Here's how the part is built. I have some questions about the finished solid (model axes, mm). Give positions to 0.01 mm unless a question says otherwise; leave off trailing zeros. Write each loop counter-clockwise with the first axis right and the second up, starting at its lowest first coordinate (ties: lowest second). Pieces come first, ordered by that corner, then holes. Notation, with made-up numbers: (8.25, -3.5) -> (19.25, -3.5) arc R23 ccw to (19.25, 13.5) -> close; hole circle Ø8 at (59, 38). An arc over 180 degrees is marked (long way). Use one line per item in the form item = value.
```python
from build123d import *

# Parameters (mm, degrees)
SKETCH1_W             = 38.1
SKETCH1_H             = 9.525
BOSS_EXTRUDE1_DEPTH   = 6.35
F_4_CLEARANCE_HOLE1_D = 3.2639


with BuildPart() as part:
    # Sketch1 → Boss-Extrude1 (new body)
    with BuildSketch(Plane(origin=(0, 0, 0), x_dir=(1, 0, 0), z_dir=(0, 1, 0))):
        Rectangle(SKETCH1_W, SKETCH1_H)
    extrude(amount=BOSS_EXTRUDE1_DEPTH)

    # #4 Clearance Hole1 (through all)
    with Locations(Plane(origin=(0, 6.35, 0), x_dir=(1, 0, 0), z_dir=(0, 1, 0))):
        with Locations((-14.2875, 0)):
            f_4_clearance_hole1 = Hole(F_4_CLEARANCE_HOLE1_D / 2)

    # Mirror1: #4 Clearance Hole1 across plane
    add(f_4_clearance_hole1.mirror(Plane(origin=(0, 0, 0), x_dir=(0, 0, 1), z_dir=(1, 0, 0))), mode=Mode.SUBTRACT)


solid = part.part
```
Q1. If we mould it in two halves opening along Z, with no side actions, what happens to faces 1 (the face through (0, 3, -4.762)), 2 (the face through (-19.05, 3, 0)), 3 (the face through (12.657, 3.131, -0.072))? For each: +Z half, -Z half, draft (parallel to the pull), parting line (faces both ways), or undercut.
Result set:
face_1 = -Z half
face_2 = draft
face_3 = undercut
Q2. I want a section at A-A, the plane z = 0. Write out the boundary of the cut face in (x, y), and give its area (3 significant figures).
Result set:
outline = (-19.05, 0) -> (-15.92, 0) -> (-15.92, 6.35) -> (-19.05, 6.35) -> close; (-12.66, 0) -> (12.66, 0) -> (12.66, 6.35) -> (-12.66, 6.35) -> close; (15.92, 0) -> (19.05, 0) -> (19.05, 6.35) -> (15.92, 6.35) -> close
area = 200 mm2
Q3. If I drill on line 1 along X through (y, z) = (1.75, 0.25); line 2 along Z through (x, y) = (-14, 1.75); line 3 along Z through (x, y) = (15.5, 6), over which ranges is the centre line in solid material (lowest first)? Write a range as from..to.
Result set:
line_1 = -19.05..-15.9, -12.67..12.67, 15.9..19.05
line_2 = -4.76..-1.61, 1.61..4.76
line_3 = -4.76..-1.09, 1.09..4.76
Q4. I want a section at B-B, the plane y = 1.75. Write out the boundary of the cut face in (x, z).
Result set:
outline = (-19.05, -4.76) -> (19.05, -4.76) -> (19.05, 4.76) -> (-19.05, 4.76) -> close; hole circle Ø3.26 at (-14.29, 0); hole circle Ø3.26 at (14.29, 0)
